CAD build for the part. Positions are in the model's coordinates, mm. A direction names the side the tool comes from. Coordinates: 2 decimals unless noted, no trailing zeros. Order: outer loops, then holes, each group sorted by start corner. A loop starts at its lowest first (then second) coordinate and runs counter-clockwise, first axis right, second up. Notation, with made-up numbers: (63, -25.75) - (88, -25.75) arc R20 ccw to (88, -18.75) - close; hole circle Ø7 at (73, 55). An arc over 180 degrees is marked (long way). Return JSON: item names as keys, results as strings.
from build123d import *

# Parameters (mm, degrees)
SKETCH1_R           = 7.5
SKETCH1_R_2         = 4
BOSS_EXTRUDE1_DEPTH = 2
SKETCH2_R           = 7
SKETCH2_R_2         = 4
BOSS_EXTRUDE2_DEPTH = 1
SKETCH3_R           = 7.5
SKETCH3_R_2         = 4
BOSS_EXTRUDE3_DEPTH = 11
SKETCH4_R           = 7
SKETCH4_R_2         = 4
BOSS_EXTRUDE4_DEPTH = 1
SKETCH5_R           = 7.5
SKETCH5_R_2         = 4
BOSS_EXTRUDE5_DEPTH = 2


with BuildPart() as part:
    # Sketch1 → Boss-Extrude1 (new body)
    with BuildSketch(Plane(origin=(0, 0, 0), x_dir=(0, 0, -1), z_dir=(1, 0, 0))):
        Circle(SKETCH1_R)
        Circle(SKETCH1_R_2, mode=Mode.SUBTRACT)
    extrude(amount=BOSS_EXTRUDE1_DEPTH)

    # Sketch2 → Boss-Extrude2 (add)
    with BuildSketch(Plane(origin=(2, 0, 0), x_dir=(0, 0, -1), z_dir=(1, 0, 0))):
        Circle(SKETCH2_R)
        Circle(SKETCH2_R_2, mode=Mode.SUBTRACT)
    extrude(amount=BOSS_EXTRUDE2_DEPTH)

    # Sketch3 → Boss-Extrude3 (add)
    with BuildSketch(Plane(origin=(3, 0, 0), x_dir=(0, 0, -1), z_dir=(1, 0, 0))):
        Circle(SKETCH3_R)
        Circle(SKETCH3_R_2, mode=Mode.SUBTRACT)
    extrude(amount=BOSS_EXTRUDE3_DEPTH)

    # Sketch4 → Boss-Extrude4 (add)
    with BuildSketch(Plane(origin=(14, 0, 0), x_dir=(0, 0, -1), z_dir=(1, 0, 0))):
        Circle(SKETCH4_R)
        Circle(SKETCH4_R_2, mode=Mode.SUBTRACT)
    extrude(amount=BOSS_EXTRUDE4_DEPTH)

    # Sketch5 → Boss-Extrude5 (add)
    with BuildSketch(Plane(origin=(15, 0, 0), x_dir=(0, 0, -1), z_dir=(1, 0, 0))):
        Circle(SKETCH5_R)
        Circle(SKETCH5_R_2, mode=Mode.SUBTRACT)
    extrude(amount=BOSS_EXTRUDE5_DEPTH)


solid = part.part
Item 1: Band-saw the part on C-C, the plane x = 14.25. List the corners of the cut face in (y, z), then the cut area to 3 significant figures.
Findings below:
{"outline": "circle Ø14 at (0, 0); hole circle Ø8 at (0, 0)", "area": "104 mm²"}
Item 2: Band-saw the part on A-A, the plane y = 0. List the corners of the cut face in (x, z).
Findings below:
{"outline": "(0, -7.5) - (2, -7.5) - (2, -7) - (3, -7) - (3, -7.5) - (14, -7.5) - (14, -7) - (15, -7) - (15, -7.5) - (17, -7.5) - (17, -4) - (0, -4) - close; (0, 4) - (17, 4) - (17, 7.5) - (15, 7.5) - (15, 7) - (14, 7) - (14, 7.5) - (3, 7.5) - (3, 7) - (2, 7) - (2, 7.5) - (0, 7.5) - close"}
Item 3: Band-saw the part on D-D, the plane z = 4.25. List the corners of the cut face in (x, y).
Findings below:
{"outline": "(0, -6.18) - (2, -6.18) - (2, -5.56) - (3, -5.56) - (3, -6.18) - (14, -6.18) - (14, -5.56) - (15, -5.56) - (15, -6.18) - (17, -6.18) - (17, 6.18) - (15, 6.18) - (15, 5.56) - (14, 5.56) - (14, 6.18) - (3, 6.18) - (3, 5.56) - (2, 5.56) - (2, 6.18) - (0, 6.18) - close"}
Item 4: Which spindle directions (+Z, -Z, +X, -X, +Y, -Y) get a long thin tool onto all of the face, cutting with end or side? Do faces 4 (the flat face through (15, 2, -7)), 5 (the cylindrical face through (0.986, 0.33, 7.493)). Say none if no direction does.
Findings below:
{"face 4": "none", "face 5": "+X, -X"}
Item 5: Mould opens along X. For faces 1 (the flat face through (3, 2, -7)), 2 (the cylindrical face through (8.381, -3.905, 0.867)), 3 (the flat face through (17, -3, -3)) say: released by +X, released by -X, zero draft, split by the parting line, or undercut.
Findings below:
{"face 1": "undercut", "face 2": "zero draft", "face 3": "released by +X"}
Item 6: Wall check: L1, parallel to Y at x = 4.75, z = 0; L2, parallel to Y at x = 1, z = 1; L3, parallel to Z at x = 5, y = 3. Give the ranges that are in metal, low to high. Write a range as [from, to].
Findings below:
{"L1": "y = [-7.5, -4], [4, 7.5]", "L2": "y = [-7.43, -3.87], [3.87, 7.43]", "L3": "z = [-6.87, -2.65], [2.65, 6.87]"}
Item 7: Drop flat-ended pins along their axis: P1, Ø1.5, axis at x = 4.5, z = 6, coming from the -Y side; P2, Ø2, axis at x = 2.5, y = -4.5, coming from the -Z side. Give the stop position or say it passes through.
Findings below:
{"P1": "stops at y = -5.36", "P2": "stops at z = -6.56"}
